Geometry check sheet. Reference: the model listing, model coordinates, mm. Face numbers are marked on the shaded views. A direction names the side the tool comes from. Coordinates: 2 decimals unless noted, no trailing zeros. Loops run counter-clockwise (first coordinate to the right, second up) from the corner with the lowest first, then second, coordinate; pieces in that order, holes last.
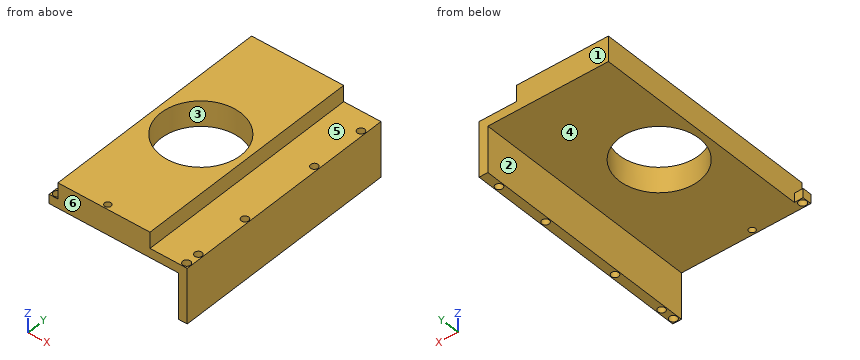
from build123d import *

# Parameters (mm, degrees)
SKETCH1_R             = 1.016
BOSS_EXTRUDE1_DEPTH   = 15.24
BOSS_EXTRUDE1_2_DEPTH = 15.24
SKETCH2_W             = 33.244360662
SKETCH2_H             = 63.5
BOSS_EXTRUDE2_DEPTH   = 2.54
SKETCH3_W             = 38.1
SKETCH3_H             = 15.24
BOSS_EXTRUDE3_DEPTH   = 2.54
SKETCH4_R             = 1.016
CUT_EXTRUDE1_DEPTH    = 41.040262237
SKETCH5_R             = 1.071714946
CUT_EXTRUDE2_DEPTH    = 41.040262237
SKETCH6_R             = 11.0000034
CUT_EXTRUDE4_DEPTH    = 41.040262237
BOSS_EXTRUDE4_START   = 4.445
SKETCH7_W             = 25.4
SKETCH7_H             = 63.5
SKETCH7_R             = 11.0000034
BOSS_EXTRUDE4_DEPTH   = 4.445
SKETCH8_W             = 35.681993508
SKETCH8_H             = 2.54
CUT_EXTRUDE5_DEPTH    = 12.7
SKETCH9_R             = 0.889
CUT_EXTRUDE6_DEPTH    = 12.7


with BuildPart() as part:
    # Sketch1 → Boss-Extrude1 (new body)
    with BuildSketch(Plane.XY):
        Polygon((19.05, 0), (19.05, 31.75), (17.840996754, 31.75), (16.631993508, 31.75), (16.631993508, -31.75), (19.05, -31.75), align=None)
        with Locations((17.840996754, -26.657844962)):
            Circle(SKETCH1_R, mode=Mode.SUBTRACT)
        with Locations((17.840996754, -11.385809707)):
            Circle(SKETCH1_R, mode=Mode.SUBTRACT)
        with Locations((17.840996754, 11.385809707)):
            Circle(SKETCH1_R, mode=Mode.SUBTRACT)
        with BuildLine():
            ThreePointArc((17.840996754, 25.641844962), (16.824996754, 26.657844962), (17.840996754, 27.673844962))
            ThreePointArc((17.840996754, 27.673844962), (18.856996754, 26.657844962), (17.840996754, 25.641844962))
        make_face(mode=Mode.SUBTRACT)
    extrude(amount=-BOSS_EXTRUDE1_DEPTH)

    # Sketch2 → Boss-Extrude2 (add)
    with BuildSketch(Plane.XY):
        with Locations((0.009813177, 0)):
            Rectangle(SKETCH2_W, SKETCH2_H)
    extrude(amount=-BOSS_EXTRUDE2_DEPTH)

    # Sketch3 → Boss-Extrude3 (add)
    with BuildSketch(Plane.XZ.offset(31.75)):
        with Locations((0, -7.62)):
            Rectangle(SKETCH3_W, SKETCH3_H)
    extrude(amount=-BOSS_EXTRUDE3_DEPTH)

    # Sketch5 → Cut-Extrude2 (cut, through all)
    with BuildSketch(Plane.XY):
        with Locations((-17.827792249, -30.48)):
            Circle(SKETCH5_R)
        with Locations((17.827792249, -30.48)):
            Circle(SKETCH5_R)
    extrude(amount=-CUT_EXTRUDE2_DEPTH, mode=Mode.SUBTRACT)

    # Sketch6 → Cut-Extrude4 (cut, through all)
    with BuildSketch(Plane.XY):
        with Locations((-3.912367154, 0)):
            Circle(SKETCH6_R)
    extrude(amount=-CUT_EXTRUDE4_DEPTH, mode=Mode.SUBTRACT)

    # Sketch7 → Boss-Extrude4 (add)
    with BuildSketch(Plane.XY.offset(BOSS_EXTRUDE4_START)):
        with Locations((-3.912367154, 0)):
            Rectangle(SKETCH7_W, SKETCH7_H)
        with Locations((-3.912367154, 0)):
            Circle(SKETCH7_R, mode=Mode.SUBTRACT)
    extrude(amount=-BOSS_EXTRUDE4_DEPTH)

    # Sketch8 → Cut-Extrude5 (cut)
    with BuildSketch(Plane(origin=(0, 0, -15.24), x_dir=(-1, 0, 0), z_dir=(0, 0, -1))):
        with Locations((1.209003246, -30.48)):
            Rectangle(SKETCH8_W, SKETCH8_H)
    extrude(amount=-CUT_EXTRUDE5_DEPTH, mode=Mode.SUBTRACT)

    # Sketch9 → Cut-Extrude6 (cut)
    with BuildSketch(Plane.XY.offset(4.445)):
        with Locations((-3.912367154, -30.48)):
            Circle(SKETCH9_R)
    extrude(amount=-CUT_EXTRUDE6_DEPTH, mode=Mode.SUBTRACT)


with BuildPart() as body_2:
    # Sketch1 → Boss-Extrude1 2 (new body)
    with BuildSketch(Plane.XY):
        with Locations((-17.840996754, -26.657844962)):
            Circle(SKETCH1_R)
    extrude(amount=-BOSS_EXTRUDE1_2_DEPTH)

    # Sketch4 → Cut-Extrude1 (cut, through all)
    with BuildSketch(Plane.XY):
        with Locations((-17.840996754, -26.657844962)):
            Circle(SKETCH4_R)
    extrude(amount=-CUT_EXTRUDE1_DEPTH, mode=Mode.SUBTRACT)


solid = part.part
(1) Sectioned sample at B-B on y = -30.48. State how many separate pieces and enclosed holes the cut face has, and give its area (3 significant figures).
Findings:
separate pieces: 4
enclosed holes: 0
area: 190 mm2
(2) Access from +Z, -Z, +X, -X, +Y, -Y to the whole of each face (thin tool, end or side, straight path). Record for the marked faces 4, 5 and 6.
Findings:
face 4: -Z, -X, +Y, -Y
face 5: +Z, +X, +Y, -Y
face 6: +Z, -Z, +X, -X, -Y
(3) Draft check along X on the marked faces 1, 2 and 3. Enter one of: +X half, -X half, draft (parallel to the pull), parting line (faces both ways), or undercut.
Findings:
face 1: draft
face 2: -X half
face 3: undercut
(4) Scan lines: L1, parallel to Z at x = -11.5, y = -28 (3 decimals); L2, parallel to X at y = 20, z = -3.5; L3, parallel to Y at x = 17, z = -0.25. Record each from-to range of solid material in increasing order.
Findings:
L1: z = -2.54 to 4.445
L2: x = 16.63 to 19.05
L3: y = -31.75 to -31.16, -29.8 to -27.23, -26.09 to -11.96, -10.82 to 10.82, 11.96 to 26.09, 27.23 to 31.75
(5) Sectioned sample at C-C on x = 3. Record the cut outline in (y, z) (3 decimals).
Findings:
outline: (-31.75, -2.54) - (-8.557, -2.54) - (-8.557, 4.445) - (-31.75, 4.445) - close; (8.557, -2.54) - (31.75, -2.54) - (31.75, 4.445) - (8.557, 4.445) - close
(6) Sectioned sample at D-D on z = 1. Record the cut outline in (x, y).
Findings:
outline: (-16.61, -31.75) - (8.79, -31.75) - (8.79, 31.75) - (-16.61, 31.75) - close; hole circle Ø22 at (-3.91, 0); hole circle Ø1.78 at (-3.91, -30.48)
(7) Sectioned sample at A-A on y = 0. Record the cut outline in (x, z) (3 decimals), and give its area (3 significant figures).
Findings:
outline: (-16.612, -2.54) - (-14.912, -2.54) - (-14.912, 4.445) - (-16.612, 4.445) - close; (7.088, -2.54) - (16.632, -2.54) - (16.632, -15.24) - (19.05, -15.24) - (19.05, 0) - (8.788, 0) - (8.788, 4.445) - (7.088, 4.445) - close
area: 80.5 mm2
(8) Gauge pin test, flat ends, axial feed: pin 1 Ø4 at (x, y) = (9, -13) entering from +Z (3 decimals); pin 2 Ø1.2 at (x, y) = (-18, -30.5) entering from +Z; pin 3 Ø3.5 at (y, z) = (14.5, 0) entering from -X; pin 4 Ø2 at (x, y) = (1.5, 8.5) entering from -Z. Record the tip position at first contact, or that the pin passes through.
Findings:
pin 1: stops at z = 4.445
pin 2: passes through
pin 3: stops at x = -16.61
pin 4: stops at z = -2.54
